Verification items for the finished model (mm, model axes). A direction names the side the tool comes from. Round coordinates to 2 decimals unless told otherwise and drop trailing zeros. Order: outer loops, then holes, each group sorted by start corner. A loop starts at its lowest first (then second) coordinate and runs counter-clockwise, first axis right, second up. Notation, with made-up numbers: (-14.75, 44.5) -> (8.25, 44.5) arc R11 ccw to (8.25, 49.5) -> close; hole circle Ø11 at (40.25, 65). An arc over 180 degrees is marked (long way). Put each result on its own line as item: value.
from build123d import *

# Parameters (mm, degrees)
CHAMFER_1_SIZE      = 1
SKETCH_2_R          = 1.25
SKETCH_2_R_2        = 1
CUT_EXTRUDE_1_DEPTH = 4
SKETCH_3_R          = 1.5
CUT_EXTRUDE_2_DEPTH = 4
SKETCH_4_R          = 6.3
CUT_EXTRUDE_3_DEPTH = 1
CUT_EXTRUDE_4_DEPTH = 0.5


with BuildPart() as part:
    # 草图1 → 旋转1 (revolve)
    with BuildSketch(Plane.XY, mode=Mode.PRIVATE) as revolve_1_sk:
        Polygon((2.25, 0), (2.25, 26), (8.3, 26), (8.3, 25), (23.5, 25), (23.5, 24), (24.5, 24), (24.5, 21), (23.5, 21), (23.5, 20.5), (24.5, 20.5), (24.5, 0), align=None)
    revolve(revolve_1_sk.sketch.rotate(Axis((0, 0, 0), (0, 1, 0)), 90), axis=Axis((0, 0, 0), (0, 1, 0)))

    # 倒角1
    chamfer_1_edges = [part.edges().sort_by_distance(p)[0] for p in [
        (0, 0, 24.5),
    ]]
    chamfer(chamfer_1_edges, length=CHAMFER_1_SIZE)

    # 草图2 → 切除-拉伸1 (cut)
    with BuildSketch(Plane(origin=(0, 25, 0), x_dir=(1, 0, 0), z_dir=(0, 1, 0))):
        with Locations(Location((13.611805538, 13.611805538, 0), (0, 0, 270))):
            Circle(SKETCH_2_R)
        with Locations(Location((13.611805538, -13.611805538, 0), (0, 0, 270))):
            Circle(SKETCH_2_R)
        with Locations(Location((-13.611805538, -13.611805538, 0), (0, 0, 270))):
            Circle(SKETCH_2_R)
        with Locations(Location((-13.611805538, 13.611805538, 0), (0, 0, 270))):
            Circle(SKETCH_2_R)
        with Locations(Location((-9.020811649, 10.377256728, 0), (0, 0, 270))):
            Circle(SKETCH_2_R_2)
        with Locations(Location((-3.326426064, -13.341566236, 0), (0, 0, 270))):
            Circle(SKETCH_2_R_2)
        with Locations(Location((9.020811649, 10.377256728, 0), (0, 0, 90))):
            Circle(SKETCH_2_R_2)
    extrude(amount=-CUT_EXTRUDE_1_DEPTH, mode=Mode.SUBTRACT)

    # 草图3 → 切除-拉伸2 (cut)
    with BuildSketch(Plane.XZ):
        with Locations(Location((0, 9.5, 0), (0, 0, 270))):
            Circle(SKETCH_3_R)
        with Locations(Location((8.838834765, 8.838834765, 0), (0, 0, 270))):
            Circle(SKETCH_3_R)
        with Locations(Location((9.5, 0, 0), (0, 0, 270))):
            Circle(SKETCH_3_R)
        with Locations(Location((8.838834765, -8.838834765, 0), (0, 0, 270))):
            Circle(SKETCH_3_R)
        with Locations(Location((0, -9.5, 0), (0, 0, 270))):
            Circle(SKETCH_3_R)
        with Locations(Location((-8.838834765, -8.838834765, 0), (0, 0, 270))):
            Circle(SKETCH_3_R)
        with Locations(Location((-9.5, 0, 0), (0, 0, 270))):
            Circle(SKETCH_3_R)
        with Locations(Location((-8.838834765, 8.838834765, 0), (0, 0, 270))):
            Circle(SKETCH_3_R)
    extrude(amount=-CUT_EXTRUDE_2_DEPTH, mode=Mode.SUBTRACT)

    # 草图4 → 切除-拉伸3 (cut)
    with BuildSketch(Plane.XZ):
        with Locations(Location((0, 0, 0), (0, 0, 270))):
            Circle(SKETCH_4_R)
    extrude(amount=-CUT_EXTRUDE_3_DEPTH, mode=Mode.SUBTRACT)

    # 草图5 → 切除-拉伸4 (cut)
    with BuildSketch(Plane(origin=(0, 25, 0), x_dir=(1, 0, 0), z_dir=(0, 1, 0))):
        with BuildLine():
            Line((-7.020811649, 10.377256728), (7.020811649, 10.377256728))
            ThreePointArc((7.020811649, 10.377256728), (7.72791843, 10.670149947), (8.020811649, 11.377256728))
            Line((8.020811649, 11.377256728), (8.020811649, 21.088833842))
            ThreePointArc((8.020811649, 21.088833842), (7.72791843, 21.795940623), (7.020811649, 22.088833842))
            Line((7.020811649, 22.088833842), (-7.020811649, 22.088833842))
            ThreePointArc((-7.020811649, 22.088833842), (-7.72791843, 21.795940623), (-8.020811649, 21.088833842))
            Line((-8.020811649, 21.088833842), (-8.020811649, 11.377256728))
            ThreePointArc((-8.020811649, 11.377256728), (-7.72791843, 10.670149947), (-7.020811649, 10.377256728))
        make_face()
    extrude(amount=-CUT_EXTRUDE_4_DEPTH, mode=Mode.SUBTRACT)


solid = part.part
Item 1: Tool access check on faces 5 (the cylindrical face through (-1.52, 13.68, 1.66)), 6 (the flat face through (14, 21, -14)), 7 (the flat face through (9, 4, -9)). Record the directions out of +Z, -Z, +X, -X, +Y, -Y that give a thin tool (end or side, any length) a straight path to the whole face; none if there is none.
Check sheet entries:
face 5: +Y, -Y
face 6: +Y
face 7: -Y
Item 2: Section check C-C on y = 13. Record the boundary of the cut face in (x, z), then the cut area to 3 significant figures.
Check sheet entries:
outline: circle Ø49 at (0, 0); hole circle Ø4.5 at (0, 0)
area: 1,870 mm^2
Item 3: Release check for a two-part mould opening along Y. For faces 1 (the cylindrical face through (-23.3, 20.75, 3.06)), 2 (the cylindrical face through (0, 2, -8)), 3 (the flat face through (13, 21, -20)), 4 (the flat face through (10, 4, 0)) record: +Y half, -Y half, draft (parallel to the pull), parting line (faces both ways), or undercut.
Check sheet entries:
face 1: undercut
face 2: draft
face 3: undercut
face 4: -Y half
Item 4: Gauge pin test, flat ends, axial feed: pin 1 Ø2 at (x, y) = (9.5, 3) entering from -Z; pin 2 Ø3.5 at (x, z) = (8.84, 8.84) entering from +Y; pin 3 Ø2.5 at (x, z) = (-8.84, -8.84) entering from -Y; pin 4 Ø2 at (x, z) = (-13.61, 13.61) entering from -Y. Record the tip position at first contact, or that the pin passes through.
Check sheet entries:
pin 1: stops at z = -22.98
pin 2: stops at y = 25
pin 3: stops at y = 4
pin 4: stops at y = 0
Item 5: Section check A-A on y = 3. State how many separate pieces and enclosed holes the cut face has, then the cut area to 3 significant figures.
Check sheet entries:
separate pieces: 1
enclosed holes: 9
area: 1,810 mm^2
Item 6: Material ranges on L1, parallel to X at y = 1.65, z = 0; L2, parallel to X at y = 2, z = 9.5; L3, parallel to Y at x = -21.5, z = 11.5, recorded low to high. Write a range as [from, to].
Check sheet entries:
L1: x = [-24.5, -11], [-8, -2.25], [2.25, 8], [11, 24.5]
L2: x = [-22.58, -10.19], [-7.49, -1.5], [1.5, 7.49], [10.19, 22.58]
L3: y = [0.88, 20.5], [21, 24]
